Work out the finished part from the listing and answer in its coordinate system (mm). Face numbers are marked on the shaded views. Round coordinates to 2 decimals unless told otherwise and drop trailing zeros. Loops run counter-clockwise (first coordinate to the right, second up) from the corner with the lowest first, then second, coordinate; pieces in that order, holes last. Notation, with made-up numbers: M 5.5,16.25 L 29.5,16.25 A25 ccw 29.5,42.25 Z; hole C 55,24 d4. An arc over 180 degrees is marked long. One line per item, written item: value.
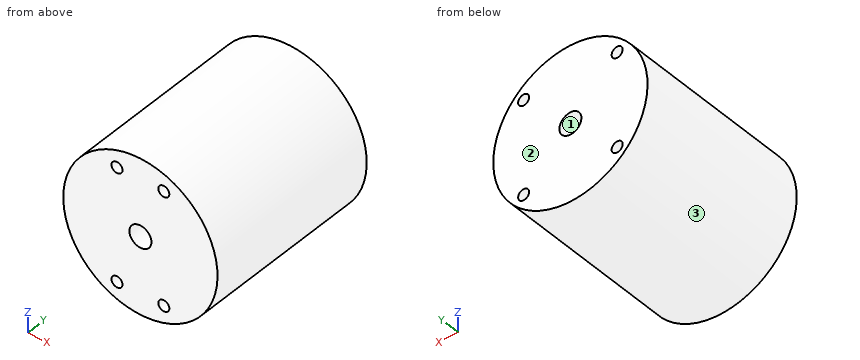
```python
from build123d import *

# Parameters (mm, degrees)
SKETCH_1_R          = 28
EXTRUDE_1_DEPTH     = 66
MM_1_D              = 4
MM_1_DEPTH          = 15
MM_1_TIP            = 1.201721238
SKETCH_5_R          = 4
CUT_EXTRUDE_1_DEPTH = 77.96752562
MM_2_D              = 4
MM_2_DEPTH          = 15
MM_2_TIP            = 1.201721238


with BuildPart() as part:
    # 草图1 → 凸台-拉伸1 (new body)
    with BuildSketch(Plane(origin=(0, 0, 0), x_dir=(1, 0, 0), z_dir=(0, 1, 0))):
        with Locations(Location((0, 0, 0), (0, 0, 270))):
            Circle(SKETCH_1_R)
    extrude(amount=EXTRUDE_1_DEPTH)

    # 大小mm 暗销孔1
    with Locations(Plane(origin=(-16.970562748, 66, -16.970562748), x_dir=(0, 0, 1), z_dir=(0, 1, 0))):
        with Locations((0, 0), (0, 33.941125496), (33.941125496, 33.941125496), (33.941125496, 0)):
            Hole(MM_1_D / 2, depth=MM_1_DEPTH)
            with Locations((0, 0, -(MM_1_DEPTH + MM_1_TIP / 2))):  # 118° drill point
                Cone(0, MM_1_D / 2, MM_1_TIP, mode=Mode.SUBTRACT)

    # 草图5 → 切除-拉伸1 (cut, through all)
    with BuildSketch(Plane(origin=(0, 66, 0), x_dir=(1, 0, 0), z_dir=(0, 1, 0))):
        with Locations(Location((0, 0, 0), (0, 0, 270))):
            Circle(SKETCH_5_R)
    extrude(amount=-CUT_EXTRUDE_1_DEPTH, mode=Mode.SUBTRACT)

    # 大小mm 暗销孔2
    with Locations(Plane(origin=(-8.5, 0, 20.5), x_dir=(0, 0, -1), z_dir=(0, -1, 0))):
        with Locations((0, 0), (0, 17), (41, 17), (41, 0)):
            Hole(MM_2_D / 2, depth=MM_2_DEPTH)
            with Locations((0, 0, -(MM_2_DEPTH + MM_2_TIP / 2))):  # 118° drill point
                Cone(0, MM_2_D / 2, MM_2_TIP, mode=Mode.SUBTRACT)


solid = part.part
```
1) Find section B-B (x = 0). Give the vertices of the cut face in (y, z), then the cut area to 3 significant figures.
Check values:
outline: M 0,-28 L 66,-28 L 66,-4 L 0,-4 Z; M 0,4 L 66,4 L 66,28 L 0,28 Z
area: 3,170 mm2
2) The mould has two halves that part along X. Classify the marked faces 1, 2 and 3: +X half, -X half, draft (parallel to the pull), parting line (faces both ways), or undercut.
Check values:
face 1: undercut
face 2: draft
face 3: parting line
3) Each of these flat-tipped pins is pushed along its axis until it touches: pin 1 (1.5 mm diameter, centred on x = -1.5, z = 1.5, fed in from -Y); pin 2 (6 mm diameter, centred on y = 38.5, z = 7.5, fed in from +X); pin 3 (8 mm diameter, centred on y = 54.5, z = -1.5, fed in from -X); pin 4 (3.5 mm diameter, centred on x = 8.5, z = -20.5, fed in from -Y). Where does it stop, or does it pass through?
Check values:
pin 1: through
pin 2: x = 27.64
pin 3: x = -28
pin 4: y = 15.15
4) Find section A-A (z = 0). Give the vertices of the cut face in (x, y), then the cut area to 3 significant figures.
Check values:
outline: M -28,0 L -4,0 L -4,66 L -28,66 Z; M 4,0 L 28,0 L 28,66 L 4,66 Z
area: 3,170 mm2
5) Find section C-C (y = 21). Give the vertices of the cut face in (x, z).
Check values:
outline: C 0,0 d56; hole C 0,0 d8
6) Find section D-D (z = -11). Give the vertices of the cut face in (x, y).
Check values:
outline: M -25.75,0 L 25.75,0 L 25.75,66 L -25.75,66 Z
7) Find the intervals of material crossed by probe 1 along Z at (x, y) = (-16, 55.5); probe 2 along X at (y, z) = (6.25, 20.5); probe 3 along Z at (x, y) = (8.5, 6), in increasing order. Write a range as from..to.
Check values:
probe 1: -22.98..-18.72, -15.22..15.22, 18.72..22.98
probe 2: -19.07..-10.5, -6.5..6.5, 10.5..19.07
probe 3: -26.68..-22.5, -18.5..18.5, 22.5..26.68
